```python
from build123d import *

# Parameters (mm, degrees)
F0_W      = 78.894876
F0_H      = 40.701952
F1_DEPTH  = 5.08
F2_R      = 5.08
F3_R      = 3.262526
F3_R_2    = 3.362851
F3_R_3    = 3.841691
F4_DEPTH  = 25.4
F5_W      = 39.447438
F5_H      = 13.209066
F6_DEPTH  = 49.53
F8_DEPTH  = 25.4
F10_DEPTH = 13.462
F11_R     = 5.989358
F12_DEPTH = 25.4


with BuildPart() as f1:
    # F0 (on Top) → F1 (new body)
    with BuildSketch(Plane.XY):
        Rectangle(F0_W, F0_H)
    extrude(amount=F1_DEPTH)

    # F2
    f2_edges = [f1.edges().sort_by_distance(p)[0] for p in [
        (-39.447438, -20.350976, 2.54),
        (39.447438, -20.350976, 2.54),
    ]]
    fillet(f2_edges, radius=F2_R)

    # F3 (on face) → F4 (cut)
    with BuildSketch(Plane.XY.offset(5.08)):
        with Locations((29.968904, 13.844252)):
            Circle(F3_R)
        with Locations((30.526463, -10.599568)):
            Circle(F3_R_2)
        with Locations((-31.362806, -10.993823)):
            Circle(F3_R_3)
    extrude(amount=-F4_DEPTH, mode=Mode.SUBTRACT)

    # F5 (on face) → F6 (join)
    with BuildSketch(Plane.XY.offset(5.08)):
        with Locations((-19.723719, 13.746443)):
            Rectangle(F5_W, F5_H)
    extrude(amount=F6_DEPTH)

    # F7 (on face) → F8 (cut)
    with BuildSketch(Plane.XZ.offset(-7.14191)):
        with BuildLine():
            Line((0, 20.121116), (0, 34.994766))
            ThreePointArc((0, 34.994766), (-10.534541, 30.641328), (-14.92249, 20.121116))
            Line((-14.92249, 20.121116), (0, 20.121116))
        make_face()
        with BuildLine():
            ThreePointArc((-14.92249, 20.121116), (-10.534541, 30.641328), (0, 34.994766))
            Line((0, 34.994766), (0, 54.61))
            Line((0, 54.61), (-14.92249, 54.61))
            Line((-14.92249, 54.61), (-14.92249, 20.121116))
        make_face()
        with BuildLine():
            ThreePointArc((-14.92249, 20.121116), (-10.569132, 9.537655), (0, 5.149625))
            Line((0, 5.149625), (0, 20.121116))
            Line((0, 20.121116), (-14.92249, 20.121116))
        make_face()
    extrude(amount=-F8_DEPTH, mode=Mode.SUBTRACT)

    # F9 (on face) → F10 (join)
    with BuildSketch(Plane.XZ.offset(-7.14191)):
        with BuildLine():
            Line((-39.447438, 54.61), (-14.92249, 54.61))
            ThreePointArc((-14.92249, 54.61), (-27.184964, 66.872474), (-39.447438, 54.61))
        make_face()
    extrude(amount=-F10_DEPTH)

    # F11 (on face) → F12 (cut)
    with BuildSketch(Plane.XZ.offset(-7.14191)):
        with Locations((-27.184964, 54.61)):
            Circle(F11_R)
    extrude(amount=-F12_DEPTH, mode=Mode.SUBTRACT)


solid = f1.part
```
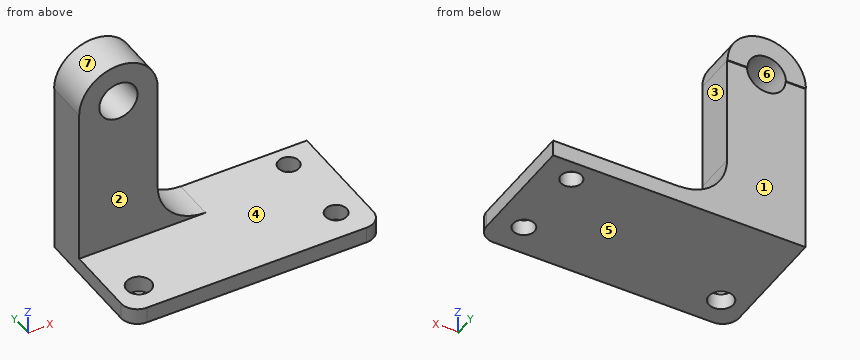
The listing builds one solid part. Answer for the finished solid, in the listing's coordinates (mm). Face numbers are marked on the shaded views. A direction names the side the tool comes from. Coordinates: 2 decimals unless noted, no trailing zeros. Write each loop counter-clockwise with the first axis right and the second up, starting at its lowest first coordinate (ties: lowest second). Pieces come first, ordered by that corner, then holes. Notation, with made-up numbers: (-32, 8.5) - (-26, 8.5) arc R15 ccw to (-26, 12.5) - close; hole circle Ø1 at (16.5, 44). An arc over 180 degrees is marked (long way). One line per item, written item: value.
1) Each of these flat-tipped pins is pushed along its axis until it touches: pin 1 Ø14.5 at (y, z) = (14.5, 30.5) entering from +X; pin 2 Ø12 at (x, y) = (7, -2) entering from +Z; pin 3 Ø12 at (x, z) = (-10.5, 41) entering from -Y. Where does it stop, or does it pass through?
Geometry check:
pin 1: stops at x = -14.92
pin 2: stops at z = 5.08
pin 3: stops at y = 7.14
2) A tool of negligible diameter and unlimited length cuts with its end or side. For the marked faces 1, 2, 3 and 4, from which of +Z, -Z, +X, -X, +Y, -Y can it reach the whole face along a straight path? Write none if from no direction.
Geometry check:
face 1: -Z, +X, -X, +Y
face 2: +Z, +X, -X, -Y
face 3: +Z, +X, +Y, -Y
face 4: +Z, +X, -Y
3) Find section D-D (x = 7.5). Give the vertices of the cut face in (y, z).
Geometry check:
outline: (-20.35, 0) - (20.35, 0) - (20.35, 5.08) - (-20.35, 5.08) - close
4) Find section A-A (y = 15). Give the vertices of the cut face in (x, z), and give its area (3 significant figures).
Geometry check:
outline: (-39.45, 0) - (26.92, 0) - (26.92, 5.08) - (0, 5.08) - (0, 5.15) arc R14.92 cw to (-14.92, 20.12) - (-14.92, 54.61) arc R12.26 ccw to (-39.45, 54.61) - close; (33.02, 0) - (39.45, 0) - (39.45, 5.08) - (33.02, 5.08) - close; hole circle Ø11.98 at (-27.18, 54.61)
area: 1,760 mm2
5) For a pull along X with two mould halves and no side action, classify the marked faces 5, 6 and 7 as pulls with the +X half, pulls with the -X half, needs draft (parallel to the pull), parting line crosses it, or undercut.
Geometry check:
face 5: needs draft
face 6: undercut
face 7: parting line crosses it
6) Find section C-C (y = 3.5). Give the vertices of the cut face in (x, z), and give its area (3 significant figures).
Geometry check:
outline: (-39.45, 0) - (39.45, 0) - (39.45, 5.08) - (-39.45, 5.08) - close
area: 401 mm2
7) Consider line 1 along X through (y, z) = (12.75, 54.61); line 2 along Z through (x, y) = (13.5, 7); line 3 along X through (y, z) = (16.5, 28.5). Determine where each line is inside the solid, lowest interval first. Write a range as from..to.
Geometry check:
line 1: x = -39.45..-33.17, -21.2..-14.92
line 2: z = 0..5.08
line 3: x = -39.45..-14.92
8) Find section B-B (x = -7). Give the vertices of the cut face in (y, z), and give its area (3 significant figures).
Geometry check:
outline: (-20.35, 0) - (20.35, 0) - (20.35, 6.89) - (7.14, 6.89) - (7.14, 5.08) - (-20.35, 5.08) - close
area: 231 mm2
